Geometry: see drawing. Coordinates: mm, zero at the bounding-box minimum. A direction names the side the tool comes from. Give positions to 0.01 mm unless a question says otherwise; leave off trailing zeros. Loops run counter-clockwise (first coordinate to the right, second up) from the corner with the lowest first, then second, coordinate; pieces in that order, holes last. Notation, with made-up numbers: (83.5, 28) - (142.5, 28) arc R28 ccw to (142.5, 56) - close; hole circle Ø2 at (53.5, -12). An arc over 180 degrees is marked (long way). One line per question, with ' | ' between items. Start each with the question number.
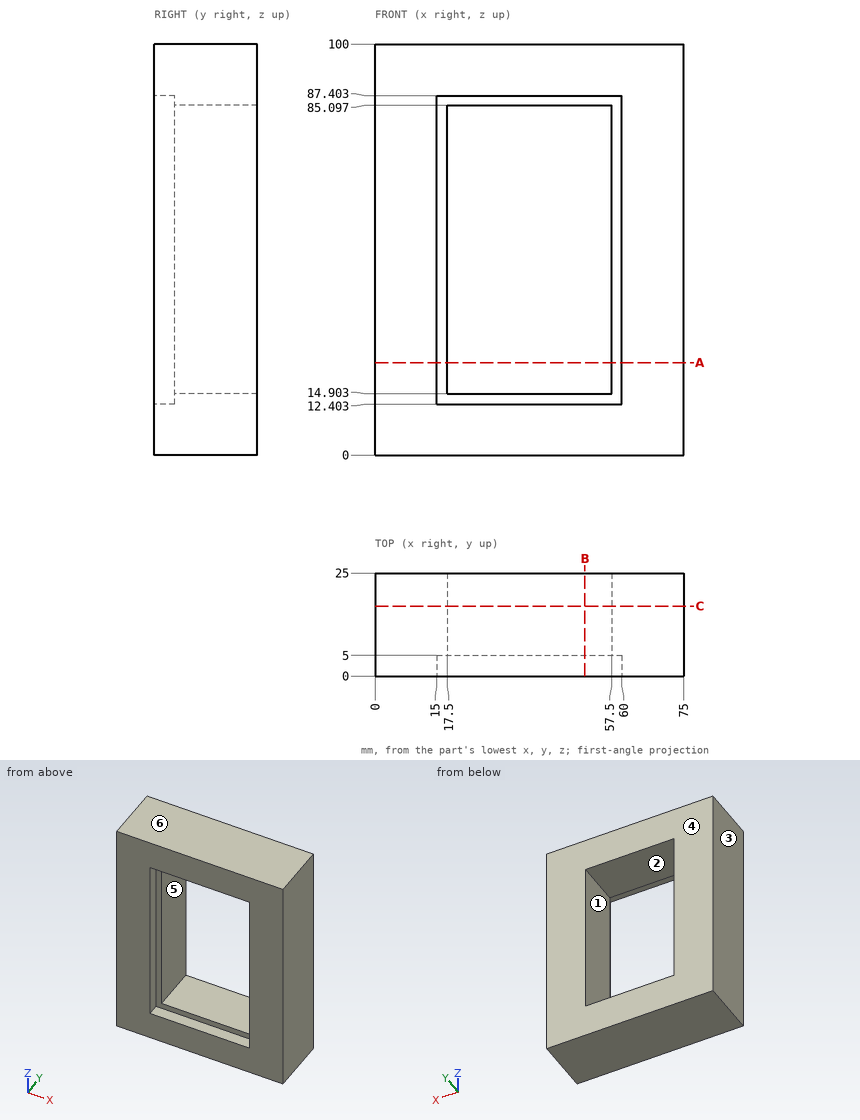
Q1. Line query: L1, parallel to Z at x = 30.5, y = 21; L2, parallel to X at y = 23.75, z = 75.5; L3, parallel to Z at x = 33.5, y = 2.5. Output: solid intervals per line, ascending. Write a range as from..to.
Q2. Access query for the marked faces 5 and 6. Directions: +Z, -Z, +X, -X, +Y, -Y. A direction counts if a zero-diameter tool reaches every point of the face in a straight line with its end or side. Return the directions, or none.
Q3. Draft query along X for the marked faces 1, 2, 3 and 4. Return one class per face: +X half, -X half, draft (parallel to the pull), parting line (faces both ways), or undercut.
Q4. Section A-A, the plane z = 22.5. Output: boundary loops of the cut face in (x, y).
Q5. Section C-C, the plane y = 17. Output: boundary loops of the cut face in (x, z).
Q6. Section B-B, the plane x = 51. Output: boundary loops of the cut face in (y, z).
Solved:
1) L1: z = 0..14.9, 85.1..100 | L2: x = 0..17.5, 57.5..75 | L3: z = 0..12.4, 87.4..100
2) face 5: +Y, -Y | face 6: +Z, +X, -X, +Y, -Y
3) face 1: undercut | face 2: undercut | face 3: -X half | face 4: draft
4) outline: (0, 0) - (15, 0) - (15, 5) - (17.5, 5) - (17.5, 25) - (0, 25) - close; (57.5, 5) - (60, 5) - (60, 0) - (75, 0) - (75, 25) - (57.5, 25) - close
5) outline: (0, 0) - (75, 0) - (75, 100) - (0, 100) - close; hole (17.5, 14.9) - (57.5, 14.9) - (57.5, 85.1) - (17.5, 85.1) - close
6) outline: (0, 0) - (25, 0) - (25, 14.9) - (5, 14.9) - (5, 12.4) - (0, 12.4) - close; (0, 87.4) - (5, 87.4) - (5, 85.1) - (25, 85.1) - (25, 100) - (0, 100) - close
